Can you work these out from the model? Positions are in its coordinate system, mm. Give positions to 0.01 mm unless a question says otherwise; leave off trailing zeros. Loops run counter-clockwise (first coordinate to the right, second up) from the corner with the lowest first, then second, coordinate; pieces in that order, holes last. Notation, with made-up numbers: (15.25, 83.25) - (51.25, 83.25) arc R24 cw to (51.25, 96.25) - close; hole circle Ø2 at (3.25, 29). An arc over 180 degrees is marked (long way). Answer as a JSON object with one key per item and string values. Group by question number.
Item 1: Please list where these lines run through material, in increasing order: L1, parallel to Z at x = 0.05, y = 334; L2, parallel to Z at x = 0.55, y = 110; L3, parallel to Z at x = 0.55, y = 188.
Item 2: Will this pin go through, and if not, where does the flat tip stop? pin 1 (3 mm diameter, centred on y = 186, z = -2, fed in from -X).
Item 3: Suppose I cut it at C-C on y = 164.5. Write out the boundary of the cut face in (x, z), and give its area (3 significant figures).
Item 4: Suppose I cut it at B-B on y = 83.5. Write out the boundary of the cut face in (x, z), and give its area (3 significant figures).
Item 5: Suppose I cut it at A-A on x = 0.4. Write out the boundary of the cut face in (y, z), and give its area (3 significant figures).
from build123d import *

# Parameters (mm, degrees)
SKETCH2_R = 0.75


with BuildPart() as part:
    # Sweep1: sweep along a path in Sketch1
    with BuildLine(Plane(origin=(0, 0, 0), x_dir=(0, 0, -1), z_dir=(1, 0, 0))) as sweep1_path:
        Line((0, 600), (0, 21.508533778))
        ThreePointArc((0, 21.508533778), (0.056650248, 20.004272941), (0.226280067, 18.508533778))
        Line((0.226280067, 18.508533778), (2.96605799, 0.45))
        ThreePointArc((2.96605799, 0.45), (0.112900451, -2.997874829), (-2.9915026, 0.225637305))
        Line((-2.9915026, 0.225637305), (-1.556649332, 19.248942344))
        ThreePointArc((-1.556649332, 19.248942344), (-1.514167351, 20.000533536), (-1.5, 20.753191044))
        Line((-1.5, 20.753191044), (-1.5, 120))
    # Sketch2 → Sweep1 (sweep)
    with BuildSketch(Plane(origin=(0, 120, 1.5), x_dir=(-1, 0, 0), z_dir=(0, 1, 0))):
        Circle(SKETCH2_R)
    sweep(path=sweep1_path.line)


solid = part.part
Worked out:
{
 "1": {"L1": "z = -0.75 to 0.75", "L2": "z = -0.51 to 0.51, 0.99 to 2.01", "L3": "z = -0.51 to 0.51"},
 "2": {"pin 1": "stops at x = -0.56"},
 "3": {"outline": "circle Ø1.5 at (0, 0)", "area": "1.77 mm2"},
 "4": {"outline": "circle Ø1.5 at (0, 0); circle Ø1.5 at (0, 1.5)", "area": "3.53 mm2"},
 "5": {"outline": "(0.18, 2.36) - (19.2, 0.92) arc R20.63 ccw to (20.75, 0.87) - (120, 0.87) - (120, 2.13) - (20.75, 2.13) arc R19.37 cw to (19.3, 2.19) - (0.27, 3.62) arc R3.63 ccw (long way) to (0.55, -3.59) - (18.6, -0.85) arc R19.37 cw to (21.51, -0.63) - (600, -0.63) - (600, 0.63) - (21.51, 0.63) arc R20.63 ccw to (18.41, 0.4) - (0.35, -2.34) arc R2.37 cw (long way) to start", "area": "926 mm2"}
}
